Could you check a few things on this model? Use its own coordinates, in mm. A direction names the side the tool comes from. Give positions to 0.01 mm unless a question says otherwise; leave off trailing zeros. Write each loop counter-clockwise with the first axis right and the second up, starting at its lowest first coordinate (ties: lowest second). Pieces come first, ordered by that corner, then holes. Notation, with made-up numbers: (77.25, -16.75) -> (106.25, -16.75) arc R14 cw to (106.25, -3.75) -> close; hole circle Ø5 at (-9.5, 84). An arc over 180 degrees is marked (long way). One line per question, with ' | ' between items.
from build123d import *

# Parameters (mm, degrees)
F2_SIZE = 12.7


with BuildPart() as f1:
    # F0 (on Front) → F1 (revolve)
    with BuildSketch(Plane.XZ):
        with BuildLine():
            Line((-25.4, 133.35), (0, 142.594844))
            Line((0, 142.594844), (0, 252.2855))
            Line((0, 252.2855), (-876.3, 252.2855))
            ThreePointArc((-876.3, 252.2855), (-885.280256, 256.005244), (-889, 264.9855))
            Line((-889, 264.9855), (-889, 412.75))
            Line((-889, 412.75), (-1270, 412.75))
            Line((-1270, 412.75), (-1270, 142.594844))
            Line((-1270, 142.594844), (-1244.6, 133.35))
            Line((-1244.6, 133.35), (-25.4, 133.35))
        make_face()
    revolve(axis=Axis((-190.5, 0, 0), (-1, 0, 0)))

    # F2
    f2_edges = [f1.edges().sort_by_distance(p)[0] for p in [
        (0, 0, -252.2855),
        (-889, 0, -412.75),
        (-1270, 0, -412.75),
    ]]
    chamfer(f2_edges, length=F2_SIZE)


solid = f1.part
Q1. Imagine slicing it at A-A on z = 0. Please give me the cut outline in (x, y).
Answer below:
outline: (-1270, -400.05) -> (-1257.3, -412.75) -> (-901.7, -412.75) -> (-889, -400.05) -> (-889, -264.99) arc R12.7 cw to (-876.3, -252.29) -> (-12.7, -252.29) -> (0, -239.59) -> (0, -142.59) -> (-25.4, -133.35) -> (-1244.6, -133.35) -> (-1270, -142.59) -> close; (-1270, 142.59) -> (-1244.6, 133.35) -> (-25.4, 133.35) -> (0, 142.59) -> (0, 239.59) -> (-12.7, 252.29) -> (-876.3, 252.29) arc R12.7 cw to (-889, 264.99) -> (-889, 400.05) -> (-901.7, 412.75) -> (-1257.3, 412.75) -> (-1270, 400.05) -> close
Q2. Imagine slicing it at C-C on x = -721. Please give me the cut outline in (y, z).
Answer below:
outline: circle Ø504.57 at (0, 0); hole circle Ø266.7 at (0, 0)
Q3. Will these pins go through, and if not, where does the flat tip stop? pin 1 (8 mm diameter, centred on x = -1091.5, y = -188.5, fed in from -Z); pin 2 (2 mm diameter, centred on x = -760.5, z = 201.5, fed in from +Y); pin 3 (10 mm diameter, centred on x = -828.5, y = 196, fed in from +Z).
Answer below:
pin 1: stops at z = -369.22 | pin 2: stops at y = 153.13 | pin 3: stops at z = 164.82
Q4. On a 3-axis mill with a long thin cutter (end or side, diameter ignored), from which of +Z, -Z, +X, -X, +Y, -Y can I reach the whole of each face in a straight line? I mean faces 1 (the conical face through (-1269.383, -153.458, 370.114)), 2 (the cylindrical face through (-450.55, 250.14, -32.84)). Say none if no direction works.
Answer below:
face 1: -X | face 2: +X
Q5. If we mould it in two halves opening along Y, with no side actions, what happens to faces 3 (the flat face through (-1270, 6, 172)), 4 (the cylindrical face through (-626.466, 40.055, 127.192)), 5 (the cylindrical face through (-1081.989, -251.152, -327.544)), 6 (the conical face through (-1245.83, -118.7, 61.74))? For each: +Y half, -Y half, draft (parallel to the pull), parting line (faces both ways), or undercut.
Answer below:
face 3: draft | face 4: undercut | face 5: parting line | face 6: undercut
Q6. If I drill on line 1 along Y through (x, z) = (-440, 0); line 2 along X through (y, z) = (-45, -343.5); line 3 along Z through (x, y) = (-384, -99.5), over which ranges is the centre line in solid material (lowest first)?
Answer below:
line 1: y = -252.29 to -133.35, 133.35 to 252.29 | line 2: x = -1270 to -889 | line 3: z = -231.84 to -88.78, 88.78 to 231.84
